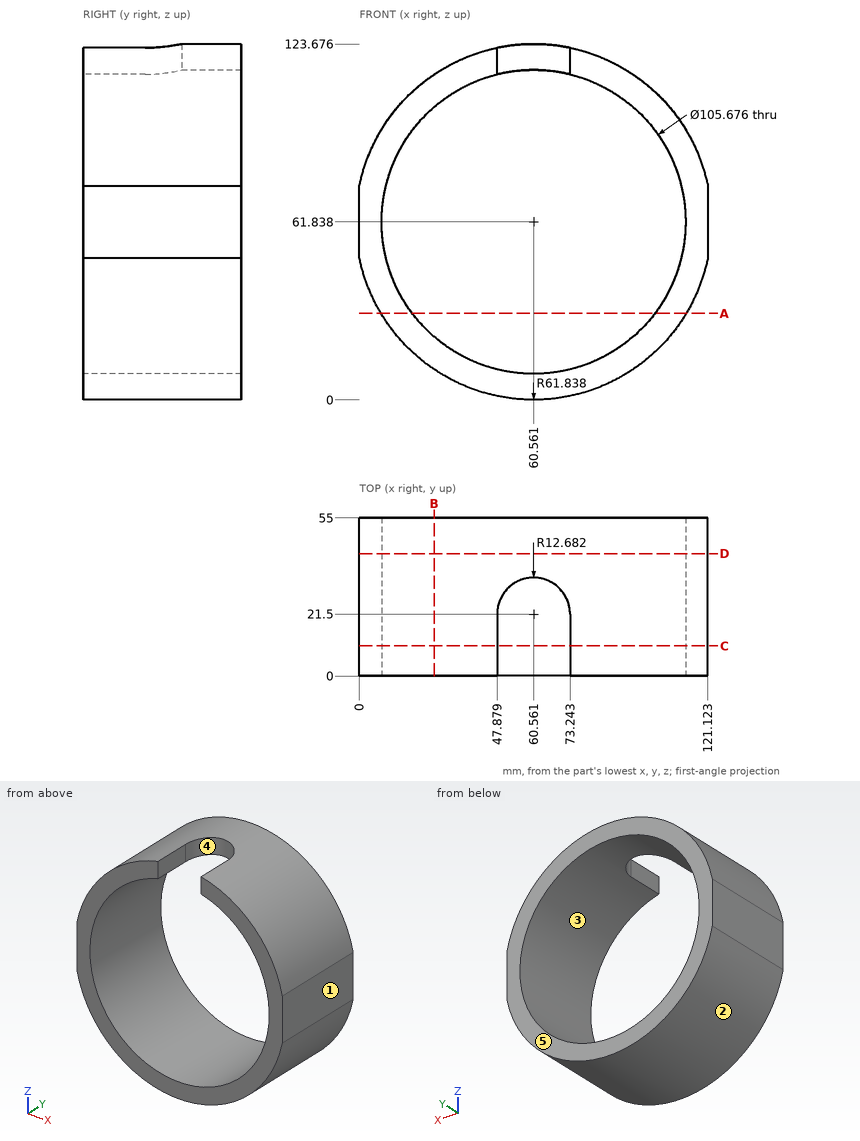
Here's the drawing with two shaded views (mm, measured from the low corner). I have some questions. A direction names the side the tool comes from. Round coordinates to 2 decimals unless told otherwise and drop trailing zeros. Write each loop counter-clockwise with the first axis right and the second up, starting at its lowest first coordinate (ties: lowest second). Pieces come first, ordered by that corner, then holes. Notation, with made-up numbers: M 67.25,87.5 L 113.25,87.5 A15 ccw 113.25,106.5 Z; hole C 0,39.5 d6. An arc over 180 degrees is marked long. Write each question's results on one line, items separated by ' | '. Start each with the question number.
1. Thinking about a two-plate mould opening in Z: for the marked faces 1, 2 and 3, which applies, +Z half, -Z half, draft (parallel to the pull), parting line (faces both ways), or undercut?
2. I'm going to push flat-ended pins straight in: pin 1 Ø2 at (x, y) = (48, 35) entering from +Z (1 decimal); pin 2 Ø12 at (x, y) = (45.5, 14) entering from -Z; pin 3 Ø7.5 at (y, z) = (8.5, 118.5) entering from +X (1 decimal). Where does each tip first touch, or does it pass through?
3. Imagine slicing it at D-D on y = 42.5. List the corners of the cut face in (x, z) for me.
4. I need wall thicknesses on L1, parallel to Z at x = 61.5, y = 45.5; L2, parallel to X at y = 28, z = 60 (1 decimal); L3, parallel to X at y = 9, z = 60.5. Which ranges of each line are inside material? Lowest first, please. Write a range as from..to.
5. Imagine slicing it at C-C on y = 10.5. List the corners of the cut face in (x, z) for me.
6. Imagine slicing it at B-B on x = 26. List the corners of the cut face in (y, z) for me (1 decimal), and give its area (3 significant figures).
7. On a 3-axis mill with a long thin cutter (end or side, diameter ignored), from which of +Z, -Z, +X, -X, +Y, -Y can I reach the whole of each face in a straight line? I mean the marked faces 4 and 5. Say none if no direction works.
8. Imagine slicing it at A-A on z = 30. List the corners of the cut face in (x, y) for me.
Result sheet:
1) face 1: draft | face 2: -Z half | face 3: undercut
2) pin 1: stops at z = 122.6 | pin 2: stops at z = 0.67 | pin 3: stops at x = 92.6
3) outline: M 0,49.34 A61.84 ccw 121.12,49.34 L 121.12,74.34 A61.84 ccw 0,74.34 Z; hole C 60.56,61.84 d105.68
4) L1: z = 0.01..9.01, 114.67..123.67 | L2: x = 0..7.8, 113.4..121.1 | L3: x = 0..7.74, 113.38..121.12
5) outline: M 0,49.34 A61.84 ccw 121.12,49.34 L 121.12,74.34 A61.84 ccw 73.24,122.36 L 73.24,113.13 A52.84 cw long 47.88,113.13 L 47.88,122.36 A61.84 ccw 0,74.34 Z
6) outline: M 0,10.6 L 55,10.6 L 55,21.9 L 0,21.9 Z; M 0,101.8 L 55,101.8 L 55,113.1 L 0,113.1 Z | area: 1,240 mm^2
7) face 4: +Z, -Y | face 5: +Z, -Z, +X, -X, +Y
8) outline: M 7.55,0 L 18.39,0 L 18.39,55 L 7.55,55 Z; M 102.73,0 L 113.57,0 L 113.57,55 L 102.73,55 Z
